```python
from build123d import *

# Parameters (mm, degrees)
F1_DEPTH    = 20
F2_R        = 2
F3_T1_DEPTH = 30
F3_T3_DEPTH = 31.2212666506
F3_T5_DEPTH = 28.9116499156
F4_R        = 5


# Not quite as in the source:
# - a fillet or chamfer that OpenCascade refuses, or shapes differently, is made with other operations: its cross-section is extruded or revolved along the edge and cut away or added


with BuildPart() as f1:
    # F0 (on Front) → F1 (new body)
    with BuildSketch(Plane.XZ):
        Polygon((-24, 29), (-24, 0), (-20, 0), (-20, 25), (20, 25), (12.4937456114, -40), (50.4937456114, -40), (55.1129790813, 0), (51.1129790813, 0), (46.9556689583, -36), (16.9556689583, -36), (24.461923347, 29), align=None)
        with BuildLine():
            Line((-20, 0), (-24, 0))
            ThreePointArc((-24, 0), (-20.3284271247, -3.8639610307), (-15, -4))
            Line((-15, -4), (-15, 0))
            Line((-15, 0), (-20, 0))
        make_face()
    extrude(amount=F1_DEPTH)

    # F2
    f2_edges = [f1.edges().sort_by_distance(p)[0] for p in [
        (-20, -10, 0),
        (-20, -10, 25),
        (16.955669, -10, -36),
        (46.955669, -10, -36),
    ]]
    fillet(f2_edges, radius=F2_R)

    # F3: fillet of radius 2 on 6 edges, made by hand

    # F3_s2 → F3_t1 (cut)
    with BuildSketch(Plane.XZ.offset(-5)):
        with BuildLine():
            ThreePointArc((-22, 29), (-23.4142135624, 28.4142135624), (-24, 27))
            Line((-24, 27), (-24, 29))
            Line((-24, 29), (-22, 29))
        make_face()
    extrude(amount=F3_T1_DEPTH, mode=Mode.SUBTRACT)

    # F3_s4 → F3_t3 (cut)
    with BuildSketch(Plane.XZ.offset(-5.6106333253)):
        with BuildLine():
            ThreePointArc((24.2044661111, 26.7705631246), (23.7107999092, 28.3306250879), (22.2176700169, 29))
            Line((22.2176700169, 29), (24.461923347, 29))
            Line((24.461923347, 29), (24.2044661111, 26.7705631246))
        make_face()
        with BuildLine():
            ThreePointArc((14.7379989415, -40), (13.2448690491, -39.3306250879), (12.7512028472, -37.7705631246))
            Line((12.7512028472, -37.7705631246), (12.4937456114, -40))
            Line((12.4937456114, -40), (14.7379989415, -40))
        make_face()
        with BuildLine():
            ThreePointArc((52.8687257512, 0), (54.3618556435, -0.6693749121), (54.8555218454, -2.2294368754))
            Line((54.8555218454, -2.2294368754), (55.1129790813, 0))
            Line((55.1129790813, 0), (52.8687257512, 0))
        make_face()
    extrude(amount=F3_T3_DEPTH, mode=Mode.SUBTRACT)

    # F3_s6 → F3_t5 (cut)
    with BuildSketch(Plane.XZ.offset(-4.4558249578)):
        with BuildLine():
            ThreePointArc((50.6982117225, -38.2294368754), (50.0420407161, -39.4931298923), (48.7114156282, -40))
            Line((48.7114156282, -40), (50.4937456114, -40))
            Line((50.4937456114, -40), (50.6982117225, -38.2294368754))
        make_face()
        with BuildLine():
            ThreePointArc((50.9085129701, -1.7705631246), (51.5646839765, -0.5068701077), (52.8953090644, 0))
            Line((52.8953090644, 0), (51.1129790813, 0))
            Line((51.1129790813, 0), (50.9085129701, -1.7705631246))
        make_face()
    extrude(amount=F3_T5_DEPTH, mode=Mode.SUBTRACT)

    # F4
    f4_edges = [f1.edges().sort_by_distance(p)[0] for p in [
        (20, -10, 25),
    ]]
    fillet(f4_edges, radius=F4_R)


solid = f1.part
```
Geometry check sheet. Reference: the model listing, model coordinates, mm. A direction names the side the tool comes from. Give positions to 0.01 mm unless a question says otherwise; leave off trailing zeros. Order: outer loops, then holes, each group sorted by start corner. A loop starts at its lowest first (then second) coordinate and runs counter-clockwise, first axis right, second up. Notation, with made-up numbers: (-16.5, 61) - (3.5, 61) arc R21 ccw to (3.5, 77) - close; hole circle Ø4 at (43, 87). An arc over 180 degrees is marked (long way). Write item = value, one per line. Start each with the question number.
1) Scan lines: L1, parallel to Z at x = 37, y = -2.5; L2, parallel to Z at x = -16, y = -2; L3, parallel to Z at x = 0.5, y = -13. Record each from-to range of solid material in increasing order.
2) Section check A-A (z = -26.5). Enter the section's corners in (x, y).
3) Gauge pin test, flat ends, axial feed: pin 1 Ø3 at (x, y) = (24, -12) entering from +Z; pin 2 Ø3 at (y, z) = (-10, -2.5) entering from +X; pin 3 Ø6 at (x, y) = (-4.5, -10) entering from -Z; pin 4 Ø5 at (y, z) = (-3, -18.5) entering from -X. Record the tip position at first contact, or that the pin passes through.
4) Access from +Z, -Z, +X, -X, +Y, -Y to the whole of each face (thin tool, end or side, straight path). Record for faces 4 (the cylindrical face through (51.545, -9.86, -0.525)), 5 (the flat face through (-15, -10, -2)), 6 (the flat face through (16.1, -9.86, -8.77)).
5) Draft check along X on faces 1 (the cylindrical face through (13.26, -9.86, -39.35)), 2 (the cylindrical face through (46.52, -10.14, -35.48)), 3 (the flat face through (31, -10, -40)). Enter one of: released by +X, released by -X, zero draft, split by the parting line, or undercut.
6) Section check B-B (y = -5.25). Enter the section's corners in (x, z).
7) Section check C-C (x = 42.5). Enter the section's corners in (y, z), then the cut area to 3 significant figures.
Geometry check:
q1.L1 = -40 to -36
q1.L2 = -4.3 to 0, 25 to 29
q1.L3 = 25 to 29
q2.outline = (14.05, -20) - (18.05, -20) - (18.05, 0) - (14.05, 0) - close; (48.05, -20) - (52.05, -20) - (52.05, 0) - (48.05, 0) - close
q3.pin_1 = 28.98
q3.pin_2 = 54.87
q3.pin_3 = 25
q3.pin_4 = 14.69
q4.face_4 = +Z, +Y, -Y
q4.face_5 = -Z, +Y, -Y
q4.face_6 = +Y, -Y
q5.face_1 = released by -X
q5.face_2 = undercut
q5.face_3 = zero draft
q6.outline = (-24, 0) arc R6.96 ccw to (-15, -4) - (-15, 0) - (-18, 0) arc R2 cw to (-20, 2) - (-20, 23) arc R2 cw to (-18, 25) - (14.39, 25) arc R5 cw to (19.36, 19.43) - (12.75, -37.77) arc R2 ccw to (14.74, -40) - (48.71, -40) arc R2 ccw to (50.7, -38.23) - (54.86, -2.23) arc R2 ccw to (52.88, 0) arc R2 ccw to (50.91, -1.77) - (47.16, -34.23) arc R2 cw to (45.17, -36) - (19.2, -36) arc R2 cw to (17.21, -33.77) - (24.2, 26.77) arc R2 ccw to (22.22, 29) - (-22, 29) arc R2 ccw to (-24, 27) - close
q7.outline = (-20, -40) - (0, -40) - (0, -36) - (-20, -36) - close
q7.area = 80.0 mm2
